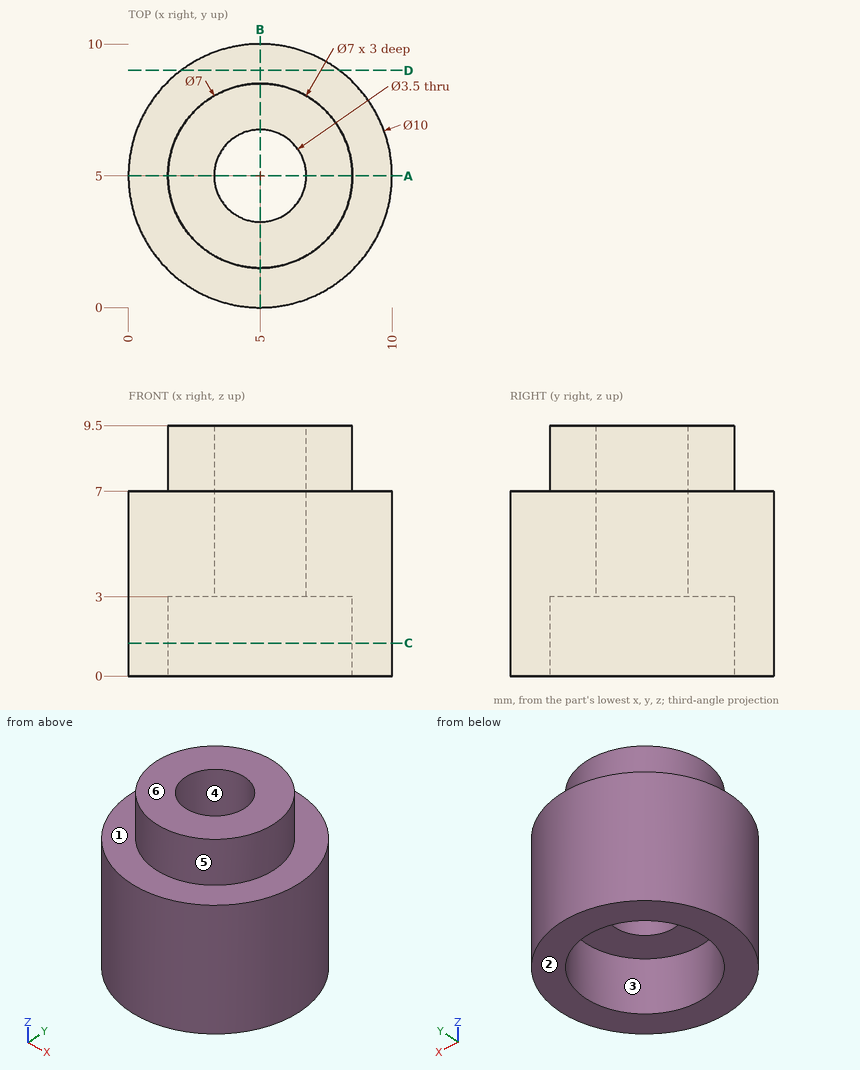
Study the drawing (mm; zero at the part's minimum x, y, z) and answer. A direction names the side the tool comes from. Coordinates: 2 decimals unless noted, no trailing zeros. Loops run counter-clockwise (first coordinate to the right, second up) from the corner with the lowest first, then second, coordinate; pieces in that order, holes last. Notation, with made-up numbers: M 68.5,-39.5 L 111.5,-39.5 A36 cw 111.5,-5.5 Z; hole C -24.5,-33.75 d10. An arc over 180 degrees is marked long. Answer in a Markdown table with one row per item.
1) Given pin 1 (5.5 mm diameter, centred on x = 3.5, y = 5, fed in from -Z); pin 2 (4 mm diameter, centred on x = 5, y = 5, fed in from -Z); pin 3 (2 mm diameter, centred on x = 1.5, z = 5.5, fed in from -Y), each flat-ended and moving along its own axis, determine where each tip first touches the part or whether it passes through.
Answers below:
| item | result |
|---|---|
| pin 1 | z = 0 |
| pin 2 | z = 3 |
| pin 3 | y = 0.67 |
2) Find section D-D (y = 9). Determine the outline of the cut face in (x, z).
Answers below:
| item | result |
|---|---|
| outline | M 2,0 L 8,0 L 8,7 L 2,7 Z |
3) Find section A-A (y = 5). Determine the outline of the cut face in (x, z).
Answers below:
| item | result |
|---|---|
| outline | M 0,0 L 1.5,0 L 1.5,3 L 3.25,3 L 3.25,9.5 L 1.5,9.5 L 1.5,7 L 0,7 Z; M 6.75,3 L 8.5,3 L 8.5,0 L 10,0 L 10,7 L 8.5,7 L 8.5,9.5 L 6.75,9.5 Z |
4) Determine the mould class of the marked faces 4, 5 and 6 for opening direction X: released by +X, released by -X, zero draft, split by the parting line, or undercut.
Answers below:
| item | result |
|---|---|
| face 4 | undercut |
| face 5 | split by the parting line |
| face 6 | zero draft |
5) Find the intervals of material crossed by probe 1 along Y at (x, z) = (5, 1.5); probe 2 along Y at (x, z) = (5, 7.75); probe 3 along Z at (x, y) = (8, 1.5), in increasing order.
Answers below:
| item | result |
|---|---|
| probe 1 | 0 to 1.5, 8.5 to 10 |
| probe 2 | 1.5 to 3.25, 6.75 to 8.5 |
| probe 3 | 0 to 7 |
6) Find section C-C (z = 1.25). Determine the outline of the cut face in (x, y), then the cut area to 3 significant figures.
Answers below:
| item | result |
|---|---|
| outline | C 5,5 d10; hole C 5,5 d7 |
| area | 40.1 mm^2 |
7) Which of the six approach directions +Z, -Z, +X, -X, +Y, -Y give full straight-line access (tool end or side, diameter ignored) to the marked faces 1, 2 and 3?
Answers below:
| item | result |
|---|---|
| face 1 | +Z |
| face 2 | -Z, +X, -X, +Y, -Y |
| face 3 | -Z |
